```python
from build123d import *

# Parameters (mm, degrees)
F1_DEPTH = 63.5
F2_DEPTH = 25.4
F3_DEPTH = 7.9375


with BuildPart() as f1:
    # F0 (on Front) → F1 (new body, symmetric)
    with BuildSketch(Plane.XZ):
        Polygon((-41.275, 9.525), (-41.275, -9.525), (41.275, -9.525), (41.275, 9.525), (22.225, 9.525), align=None)
    extrude(amount=F1_DEPTH, both=True)

    # F0 (on Front) → F2 (join, symmetric)
    with BuildSketch(Plane.XZ):
        with BuildLine():
            Line((22.225, 9.525), (41.275, 9.525))
            Line((41.275, 9.525), (41.275, 27.0002))
            ThreePointArc((41.275, 27.0002), (45.9246798487, 38.2255201513), (57.15, 42.8752))
            Line((57.15, 42.8752), (60.325, 42.8752))
            Line((60.325, 42.8752), (60.325, 61.9252))
            Line((60.325, 61.9252), (57.15, 61.9252))
            ThreePointArc((57.15, 61.9252), (56.1396828134, 61.9105836155), (55.1302112781, 61.8667466962))
            add(Edge.make_bspline(
                [(52.1201627653, 61.5611080088), (53.4052318072, 61.69652188), (54.4228886403, 61.7953477122), (55.1302112781, 61.8667466962)],
                knots=[0.8216641419, 0.8216641419, 0.8216641419, 0.8216641419, 0.8804984928, 0.8804984928, 0.8804984928, 0.8804984928], degree=3))
            ThreePointArc((52.1201627653, 61.5611080088), (30.7357738101, 49.8484883339), (22.225, 27.0002))
            Line((22.225, 27.0002), (22.225, 9.525))
        make_face()
    extrude(amount=F2_DEPTH, both=True)

    # F0 (on Front) → F3 (join, symmetric)
    with BuildSketch(Plane.XZ):
        with BuildLine():
            add(Edge.make_bspline(
                [(-41.275, 9.525), (-35.930112491, 50.6426220419), (34.1732467865, 59.6699556353), (52.1201627653, 61.5611080088)],
                knots=[0, 0, 0, 0, 0.8216641419, 0.8216641419, 0.8216641419, 0.8216641419], degree=3))
            Line((-41.275, 9.525), (22.225, 9.525))
            Line((22.225, 9.525), (22.225, 27.0002))
            ThreePointArc((22.225, 27.0002), (30.7357738101, 49.8484883339), (52.1201627653, 61.5611080088))
        make_face()
    extrude(amount=F3_DEPTH, both=True)


solid = f1.part
```
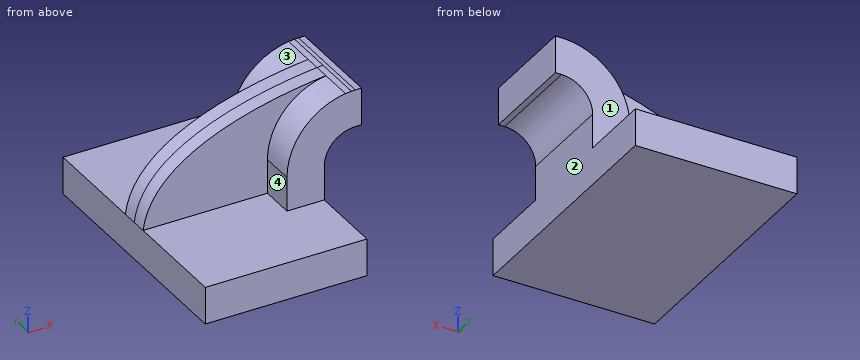
Source: CAD feature listing. Evaluate the final solid. Frame: model axes, mm. Face numbers are marked on the shaded views. A direction names the side the tool comes from. Round coordinates to 2 decimals unless told otherwise and drop trailing zeros. Loops run counter-clockwise (first coordinate to the right, second up) from the corner with the lowest first, then second, coordinate; pieces in that order, holes last. Notation, with made-up numbers: M 15.25,76 L 27.25,76 A15 cw 27.25,85 Z; hole C 59,-16.5 d10. An arc over 180 degrees is marked long. Use a Markdown table: item, result. Add a question column.
1. Set-up query: the marked faces 1, 2, 3 and 4. Return all of +Z, -Z, +X, -X, +Y, -Y with unobstructed straight access to the full face (end or side cutting, diameter ignored); none if empty.
2. Cut plane A-A, the plane z = -1. Output: boundary loops of the cut face in (x, y) (3 decimals), and give its area (3 significant figures).
3. Ray query, line 1 along Z through (x, y) = (7.5, 58) (3 decimals); line 2 along Y through (x, z) = (-15.5, 27); line 3 along X through (y, z) = (-14, 18.5) (3 decimals). Return the intervals inside material, ascending. Write a range as [from, to].
4. Cut plane B-B, the plane y = -35. Output: boundary loops of the cut face in (x, z) (3 decimals), and give its area (3 significant figures).
5. Contact query for flat-ended pins moving along their axis: pin 1 (5 mm diameter, centred on y = -2, z = 31.5, fed in from +X); pin 2 (6 mm diameter, centred on x = 23.5, y = 16, fed in from +Z); pin 3 (2 mm diameter, centred on x = -9, y = 16, fed in from +Z) (3 decimals). Output: stop coordinate, or through.
Solution:
| question | item | result |
|---|---|---|
| 1 | face 1 | +Z, +X, -X, +Y |
| 1 | face 2 | -Z, +X, +Y, -Y |
| 1 | face 3 | +Z, -X, +Y |
| 1 | face 4 | +Z, -X, -Y |
| 2 | outline | M -41.275,-63.5 L 41.275,-63.5 L 41.275,63.5 L -41.275,63.5 Z |
| 2 | area | 10,500 mm2 |
| 3 | line 1 | z = [-9.525, 9.525] |
| 3 | line 2 | y = [-7.94, 7.94] |
| 3 | line 3 | x = [22.225, 41.275] |
| 4 | outline | M -41.275,-9.525 L 41.275,-9.525 L 41.275,9.525 L -41.275,9.525 Z |
| 4 | area | 1,570 mm2 |
| 5 | pin 1 | stops at x = 42.9 |
| 5 | pin 2 | stops at z = 43.74 |
| 5 | pin 3 | stops at z = 9.525 |
